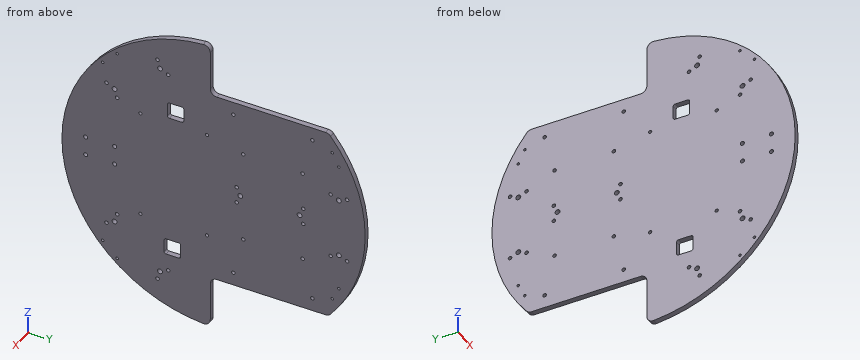
from build123d import *

# Parameters (mm, degrees)
SKETCH_1_R           = 230
EXTRUDE_1_DEPTH      = 8
SKETCH_2_W           = 80
SKETCH_2_H           = 200
CUT_EXTRUDE_1_DEPTH  = 12
SKETCH_3_R           = 2.75
CUT_EXTRUDE_2_DEPTH  = 12
SKETCH_4_R           = 3.15
CUT_EXTRUDE_3_DEPTH  = 12
SKETCH_5_R           = 3.75
SKETCH_5_R_2         = 2.75
CUT_EXTRUDE_4_DEPTH  = 10
FILLET_1_R           = 10
SKETCH_6_W           = 25
SKETCH_6_H           = 25
CUT_EXTRUDE_5_DEPTH  = 10
SKETCH_7_R           = 2.5
CUT_EXTRUDE_6_DEPTH  = 10
SKETCH_8_W           = 25
SKETCH_8_H           = 25
CUT_EXTRUDE_7_DEPTH  = 10
FILLET_3_R           = 3
SKETCH_10_R          = 2
CUT_EXTRUDE_9_DEPTH  = 326.005785815
SKETCH_11_R          = 2
CUT_EXTRUDE_10_DEPTH = 25
FILLET_4_R           = 3


with BuildPart() as part:
    # 草图1 → 凸台-拉伸1 (new body)
    with BuildSketch(Plane(origin=(0, 0, 0), x_dir=(0, 0, -1), z_dir=(1, 0, 0))):
        Circle(SKETCH_1_R)
    extrude(amount=EXTRUDE_1_DEPTH)

    # 草图2 → 切除-拉伸1 (cut)
    with BuildSketch(Plane(origin=(8, 0, 0), x_dir=(0, 0, -1), z_dir=(1, 0, 0))):
        with Locations((-190, 95)):
            Rectangle(SKETCH_2_W, SKETCH_2_H)
        with Locations((190, 95)):
            Rectangle(SKETCH_2_W, SKETCH_2_H)
    extrude(amount=-CUT_EXTRUDE_1_DEPTH, mode=Mode.SUBTRACT)

    # 草图3 → 切除-拉伸2 (cut)
    with BuildSketch(Plane(origin=(8, 0, 0), x_dir=(0, 0, -1), z_dir=(1, 0, 0))):
        with Locations((-130, 150)):
            Circle(SKETCH_3_R)
        with Locations((-130, 30)):
            Circle(SKETCH_3_R)
        with Locations((130, 30)):
            Circle(SKETCH_3_R)
        with Locations((130, 150)):
            Circle(SKETCH_3_R)
        with Locations((-70, 135)):
            Circle(SKETCH_3_R)
        with Locations((-70, 45)):
            Circle(SKETCH_3_R)
        with Locations((70, 135)):
            Circle(SKETCH_3_R)
        with Locations((70, 45)):
            Circle(SKETCH_3_R)
    extrude(amount=-CUT_EXTRUDE_2_DEPTH, mode=Mode.SUBTRACT)

    # 草图4 → 切除-拉伸3 (cut)
    with BuildSketch(Plane(origin=(8, 0, 0), x_dir=(0, 0, -1), z_dir=(1, 0, 0))):
        with Locations((-14.5, -150)):
            Circle(SKETCH_4_R)
        with Locations((14.5, -150)):
            Circle(SKETCH_4_R)
        with Locations((14.5, -194)):
            Circle(SKETCH_4_R)
        with Locations((-14.5, -194)):
            Circle(SKETCH_4_R)
    extrude(amount=-CUT_EXTRUDE_3_DEPTH, mode=Mode.SUBTRACT)

    # 草图5 → 切除-拉伸4 (cut)
    with BuildSketch(Plane(origin=(8, 0, 0), x_dir=(0, 0, -1), z_dir=(1, 0, 0))):
        with Locations((166.813442197, -81.229769803)):
            Circle(SKETCH_5_R)
        with Locations((108.962557326, -150.173769684)):
            Circle(SKETCH_5_R)
        with Locations((-108.962557326, -150.173769684)):
            Circle(SKETCH_5_R)
        with Locations((-166.813442197, -81.229769803)):
            Circle(SKETCH_5_R)
        with Locations((-45, 190)):
            Circle(SKETCH_5_R)
        with Locations((45, 190)):
            Circle(SKETCH_5_R)
        with Locations((-12.5, 35)):
            Circle(SKETCH_5_R_2)
        with Locations((12.5, 35)):
            Circle(SKETCH_5_R_2)
        with Locations((95.851669933, -146.352169)):
            Circle(SKETCH_5_R_2)
        with Locations((160.773218512, -68.981680245)):
            Circle(SKETCH_5_R_2)
        with Locations((179.92432959, -85.051370487)):
            Circle(SKETCH_5_R_2)
        with Locations((115.002781011, -162.421859242)):
            Circle(SKETCH_5_R_2)
        with Locations((-179.92432959, -85.051370487)):
            Circle(SKETCH_5_R_2)
        with Locations((-160.773218512, -68.981680245)):
            Circle(SKETCH_5_R_2)
        with Locations((-95.851669933, -146.352169)):
            Circle(SKETCH_5_R_2)
        with Locations((-115.002781011, -162.421859242)):
            Circle(SKETCH_5_R_2)
        with Locations((50.5, 202.5)):
            Circle(SKETCH_5_R_2)
        with Locations((-50.5, 202.5)):
            Circle(SKETCH_5_R_2)
        with Locations((50.5, 177.5)):
            Circle(SKETCH_5_R_2)
        with Locations((-50.5, 177.5)):
            Circle(SKETCH_5_R_2)
        with Locations((12.5, 136)):
            Circle(SKETCH_5_R_2)
        with Locations((-12.5, 136)):
            Circle(SKETCH_5_R_2)
        with Locations((0, 130.5)):
            Circle(SKETCH_5_R)
        with Locations((0, 40.5)):
            Circle(SKETCH_5_R)
    extrude(amount=-CUT_EXTRUDE_4_DEPTH, mode=Mode.SUBTRACT)

    # 圆角1
    fillet_1_edges = [part.edges().sort_by_distance(p)[0] for p in [
        (4, 174.355957742, -150),
        (4, -5, -150),
        (4, -5, -229.945645751),
        (4, 174.355957742, 150),
        (4, -5, 229.945645751),
        (4, -5, 150),
    ]]
    fillet(fillet_1_edges, radius=FILLET_1_R)

    # 草图6 → 切除-拉伸5 (cut)
    with BuildSketch(Plane(origin=(8, 0, 0), x_dir=(0, 0, -1), z_dir=(1, 0, 0))):
        with Locations((-102.5, -57.5)):
            Rectangle(SKETCH_6_W, SKETCH_6_H)
    extrude(amount=-CUT_EXTRUDE_5_DEPTH, mode=Mode.SUBTRACT)

    # 草图7 → 切除-拉伸6 (cut)
    with BuildSketch(Plane(origin=(8, 0, 0), x_dir=(0, 0, -1), z_dir=(1, 0, 0))):
        with Locations((82.5, -10)):
            Circle(SKETCH_7_R)
        with Locations((82.5, -111)):
            Circle(SKETCH_7_R)
        with Locations((-82.5, -10)):
            Circle(SKETCH_7_R)
        with Locations((-82.5, -111)):
            Circle(SKETCH_7_R)
    extrude(amount=-CUT_EXTRUDE_6_DEPTH, mode=Mode.SUBTRACT)

    # 草图8 → 切除-拉伸7 (cut)
    with BuildSketch(Plane(origin=(8, 0, 0), x_dir=(0, 0, -1), z_dir=(1, 0, 0))):
        with Locations((122.5, -62.5)):
            Rectangle(SKETCH_8_W, SKETCH_8_H)
    extrude(amount=-CUT_EXTRUDE_7_DEPTH, mode=Mode.SUBTRACT)

    # 圆角3
    fillet_3_edges = [part.edges().sort_by_distance(p)[0] for p in [
        (4, -75, -110),
        (4, -50, -110),
        (4, -50, -135),
        (4, -75, -135),
    ]]
    fillet(fillet_3_edges, radius=FILLET_3_R)

    # 草图10 → 切除-拉伸9 (cut, through all)
    with BuildSketch(Plane(origin=(8, 0, 0), x_dir=(0, 0, -1), z_dir=(1, 0, 0))):
        with Locations((168.30023639, -146.301163465)):
            Circle(SKETCH_10_R)
        with Locations((146.301163465, -168.30023639)):
            Circle(SKETCH_10_R)
        with Locations(Location((-146.301163465, -168.30023639, 0), (0, 0, 180))):
            Circle(SKETCH_10_R)
        with Locations(Location((-168.30023639, -146.301163465, 0), (0, 0, 180))):
            Circle(SKETCH_10_R)
    extrude(amount=-CUT_EXTRUDE_9_DEPTH, mode=Mode.SUBTRACT)

    # 草图11 → 切除-拉伸10 (cut)
    with BuildSketch(Plane(origin=(8, 0, 0), x_dir=(0, 0, -1), z_dir=(1, 0, 0))):
        with Locations((100, 190)):
            Circle(SKETCH_11_R)
        with Locations((120, 180)):
            Circle(SKETCH_11_R)
        with Locations((-120, 180)):
            Circle(SKETCH_11_R)
        with Locations((-100, 190)):
            Circle(SKETCH_11_R)
    extrude(amount=-CUT_EXTRUDE_10_DEPTH, mode=Mode.SUBTRACT)

    # 圆角4
    fillet_4_edges = [part.edges().sort_by_distance(p)[0] for p in [
        (4, -70, 115),
        (4, -45, 115),
        (4, -45, 90),
        (4, -70, 90),
    ]]
    fillet(fillet_4_edges, radius=FILLET_4_R)


solid = part.part
Could you check a few things on this model? Use its own coordinates, in mm. Coordinates: 2 decimals unless noted, no trailing zeros. Loops run counter-clockwise (first coordinate to the right, second up) from the corner with the lowest first, then second, coordinate; pieces in that order, holes last. Notation, with made-up numbers: (-18.75, -32) -> (39.25, -32) arc R26 cw to (39.25, -10) -> close; hole circle Ø6 at (80.25, 59.25). An arc over 180 degrees is marked (long way). Answer in a Markdown table with one row per item.
(1) Imagine slicing it at A-A (y = 112). List the corners of the cut face in (x, z) for me, plus the area to 3 significant figures.
Results found:
| item | result |
|---|---|
| outline | (0, -150) -> (8, -150) -> (8, 150) -> (0, 150) -> close |
| area | 2,400 mm^2 |
(2) Will these pins go through, and if not, where does the flat tip stop? pin 1 Ø4.5 at (y, z) = (-162.42, 115) entering from +X; pin 2 Ø4 at (x, z) = (3, 11.5) entering from -Y; pin 3 Ø4 at (x, y) = (5, -61.5) entering from +Z.
Results found:
| item | result |
|---|---|
| pin 1 | passes through |
| pin 2 | stops at y = -229.8 |
| pin 3 | stops at z = 222.17 |
(3) Imagine slicing it at B-B (x = 3.5). Give the number of separate pieces and of enclosed holes in the cut face, plus the area to 3 significant figures.
Results found:
| item | result |
|---|---|
| separate pieces | 1 |
| enclosed holes | 50 |
| area | 144,000 mm^2 |
(4) If I drill on probe 1 along Y at (x, z) = (3.5, 70); probe 2 along Y at (x, z) = (2, 82.5); probe 3 along Z at (x, y) = (0.75, 36.5), over which ranges is the centre line in solid material (lowest first)?
Results found:
| item | result |
|---|---|
| probe 1 | y = -219.09 to 42.25, 47.75 to 132.25, 137.75 to 219.09 |
| probe 2 | y = -214.69 to -113.5, -108.5 to -12.5, -7.5 to 214.69 |
| probe 3 | z = -150 to -14.8, -10.2 to 10.2, 14.8 to 150 |
